Build history of the part. All positions in model axes, mm. A direction names the side the tool comes from. Give positions to 0.01 mm unless a question says otherwise; leave off trailing zeros. Write each loop counter-clockwise with the first axis right and the second up, starting at its lowest first coordinate (ties: lowest second). Pieces come first, ordered by that corner, then holes. Notation, with made-up numbers: (0.25, 80.25) -> (55.25, 80.25) arc R21 ccw to (55.25, 95.25) -> close; hole circle Ø8 at (-30, -15.75). An arc over 180 degrees is marked (long way). Put each result on its own line as item: value. Start each with the question number.
Item 1: Slice it at D-D, the plane y = 0. Give the number of separate pieces and of enclosed holes in the cut face, plus the area to 3 significant figures.
Item 2: Two-plate mould, pull along Y, no slides. Class faces 4 (the cylindrical face through (17.1, 28.84, 0.37)), 5 (the flat face through (13.048, 2, -22)), 6 (the cylindrical face through (16.992, -5.077, 38.668)): pulls with the +Y half, pulls with the -Y half, needs draft (parallel to the pull), parting line crosses it, or undercut.
Item 3: Slice it at B-B, the plane y = 30.5. List the corners of the cut face in (x, z).
Item 4: Tool access for faces 1 (the flat face through (21.048, -11.4, -34.5)), 2 (the cylindrical face through (20.77, 13.17, 20.66)), 3 (the flat face through (13.614, 7, -22)): list every direction of +Z, -Z, +X, -X, +Y, -Y with a clear straight run to the whole face (end or side of a thin tool).
Item 5: Slice it at A-A, the plane x = 19. List the corners of the cut face in (y, z).
Item 6: Flat gauge pins, fed straight in: pin 1 Ø10 at (y, z) = (21, -2.5) entering from +X; pin 2 Ø3 at (x, z) = (16, 10) entering from +Y; pin 3 Ø3 at (y, z) = (0, -30.5) entering from -X; pin 4 Ø2 at (x, y) = (15, 14) entering from -Z. Where does each tip first touch, or does it go through?
Item 7: Drill centre lines: line 1 along Z through (x, y) = (16, 0); line 2 along Z through (x, y) = (14.75, -3.5); line 3 along Z through (x, y) = (15, 10). Where is each one in solid material? Low to high.
```python
from build123d import *

# Parameters (mm, degrees)
M3_CLEARANCE_HOLE1_D     = 3.4
M3_CLEARANCE_HOLE1_DEPTH = 8
M3_CLEARANCE_HOLE1_TIP   = 1.021463052


with BuildPart() as part:
    # Sketch1 → Revolve17 (revolve)
    with BuildSketch(Plane.XY):
        Polygon((20.481671209, 24.5), (21.047671209, 24.5), (21.047671209, 34), (20.380671209, 34), (20.380671209, 36), (21.047671209, 36), (21.047671209, 39), (13.047671209, 39), (13.047671209, 36), (13.714671209, 36), (13.714671209, 34), (13.047671209, 34), (13.047671209, 24.5), (13.613671209, 24.5), (13.613671209, 22.6), (13.047671209, 22.6), (13.047671209, 21.6), (21.047671209, 21.6), (21.047671209, 22.6), (20.481671209, 22.6), align=None)
    revolve(axis=Axis((-801.920554309, 0, 0), (1, 0, 0)))

    # M3 Clearance Hole1
    with Locations(Plane.ZY.offset(-13.047671209)):
        with Locations((0, -30.5), (0, 30.5), (30.5, 0), (-30.5, 0)):
            Hole(M3_CLEARANCE_HOLE1_D / 2, depth=M3_CLEARANCE_HOLE1_DEPTH)
            with Locations((0, 0, -(M3_CLEARANCE_HOLE1_DEPTH + M3_CLEARANCE_HOLE1_TIP / 2))):  # 118° drill point
                Cone(0, M3_CLEARANCE_HOLE1_D / 2, M3_CLEARANCE_HOLE1_TIP, mode=Mode.SUBTRACT)


solid = part.part
```
Values follow:
1. separate pieces: 4
1. enclosed holes: 0
1. area: 214 mm2
2. face 4: undercut
2. face 5: needs draft
2. face 6: parting line crosses it
3. outline: (13.05, -24.31) -> (21.05, -24.31) -> (21.05, -19.12) -> (20.38, -19.12) -> (20.38, -15.02) -> (21.05, -15.02) -> (21.05, -1.7) -> (13.05, -1.7) -> (13.05, -15.02) -> (13.71, -15.02) -> (13.71, -19.12) -> (13.05, -19.12) -> close; (13.05, 1.7) -> (21.05, 1.7) -> (21.05, 15.02) -> (20.38, 15.02) -> (20.38, 19.12) -> (21.05, 19.12) -> (21.05, 24.31) -> (13.05, 24.31) -> (13.05, 19.12) -> (13.71, 19.12) -> (13.71, 15.02) -> (13.05, 15.02) -> close
4. face 1: +Z, -Z, +X, +Y, -Y
4. face 2: +X
4. face 3: -X
5. outline: circle Ø78 at (0, 0); hole circle Ø3.4 at (-30.5, 0); hole circle Ø43.2 at (0, 0); hole circle Ø3.4 at (0, -30.5); hole circle Ø3.4 at (0, 30.5); hole circle Ø3.4 at (30.5, 0)
6. pin 1: x = 21.05
6. pin 2: y = 38.06
6. pin 3: through
6. pin 4: z = -36.77
7. line 1: -39 to -32.2, -28.8 to -21.6, 21.6 to 28.8, 32.2 to 39
7. line 2: -38.84 to -21.31, 21.31 to 38.84
7. line 3: -37.7 to -19.15, 19.15 to 37.7
